```python
from build123d import *

# Parameters (mm, degrees)
SKETCH1_W               = 54.61
SKETCH1_H               = 47.244
SKETCH1_W_2             = 41.91
SKETCH1_H_2             = 21.844
BOSS_EXTRUDE1_DEPTH     = 5.08
SKETCH2_R               = 0.93599
CUT_EXTRUDE1_DEPTH      = 73.388217522
SKETCH10_W              = 14.41958
SKETCH10_H              = 19.49958
SKETCH10_R              = 0.635
BOSS_EXTRUDE4_DEPTH     = 5.08
SKETCH11_R              = 0.635
SKETCH11_W              = 3.302
SKETCH11_H              = 76.2
BOSS_EXTRUDE5_DEPTH     = 5.08
SKETCH12_W              = 60.452
SKETCH12_H              = 6.35
SKETCH12_W_2            = 59.182
CUT_EXTRUDE2_DEPTH      = 95.448366629
SKETCH13_W              = 7.0195552
SKETCH13_H              = 78.993394517
BOSS_EXTRUDE6_DEPTH     = 4.826
FILLET1_R               = 2.54
CUT_EXTRUDE3_DEPTH      = 95.448366629
SKETCH15_W              = 9.078627065
SKETCH15_H              = 34.544
BOSS_EXTRUDE7_DEPTH     = 5.08
SKETCH16_W              = 10.16
SKETCH16_H              = 12.7
BOSS_EXTRUDE8_DEPTH     = 10.16
SKETCH17_R              = 0.635
CUT_EXTRUDE4_DEPTH      = 71.364025147
SKETCH18_W              = 10.16
SKETCH18_H              = 6.35
BOSS_EXTRUDE9_DEPTH     = 12.76096
CUT_EXTRUDE5_DEPTH      = 73.410049688
CUT_EXTRUDE5_DEPTH_BACK = 73.410049688
SKETCH19_R              = 0.635
SKETCH20_W              = 10.16
SKETCH20_H              = 6.35
BOSS_EXTRUDE10_DEPTH    = 6.28904
CUT_EXTRUDE7_DEPTH      = 19.05


with BuildPart() as part:
    # Sketch1 → Boss-Extrude1 (new body)
    with BuildSketch(Plane.XY):
        with Locations((27.305, 23.622)):
            Rectangle(SKETCH1_W, SKETCH1_H)
        with Locations((27.305, 23.622)):
            Rectangle(SKETCH1_W_2, SKETCH1_H_2, mode=Mode.SUBTRACT)
    extrude(amount=BOSS_EXTRUDE1_DEPTH)

    # Sketch2 → Cut-Extrude1 (cut, through all)
    with BuildSketch(Plane.XY.offset(5.08)):
        with Locations((2.80543, 28.62199)):
            Circle(SKETCH2_R)
        with Locations((2.80543, 18.62201)):
            Circle(SKETCH2_R)
        with Locations((51.80457, 28.62199)):
            Circle(SKETCH2_R)
        with Locations((51.80457, 18.62201)):
            Circle(SKETCH2_R)
    extrude(amount=-CUT_EXTRUDE1_DEPTH, mode=Mode.SUBTRACT)

    # Sketch10 → Boss-Extrude4 (add)
    with BuildSketch(Plane.XY.offset(5.08)):
        with Locations((61.81979, 23.622)):
            Rectangle(SKETCH10_W, SKETCH10_H)
        with Locations((64.35979, 21.49221)):
            Circle(SKETCH10_R, mode=Mode.SUBTRACT)
        with Locations((64.35979, 25.75179)):
            Circle(SKETCH10_R, mode=Mode.SUBTRACT)
    extrude(amount=-BOSS_EXTRUDE4_DEPTH)

    # Sketch11 → Boss-Extrude5 (add)
    with BuildSketch(Plane.XY.offset(5.08)):
        Polygon((0, 47.244), (-5.842, 47.244), (-5.842, 64.262), (-15.748, 64.262), (-15.748, -17.018), (-4.572, -17.018), (-4.572, 0), (0, 0), align=None)
        with Locations(Location((-4.572, 21.49221, 0), (0, 0, 180))):
            Circle(SKETCH11_R, mode=Mode.SUBTRACT)
        with Locations(Location((-4.572, 25.75179, 0), (0, 0, 180))):
            Circle(SKETCH11_R, mode=Mode.SUBTRACT)
        with Locations((-10.795, 23.622)):
            Rectangle(SKETCH11_W, SKETCH11_H, mode=Mode.SUBTRACT)
    extrude(amount=-BOSS_EXTRUDE5_DEPTH)

    # Sketch12 → Cut-Extrude2 (cut, through all)
    with BuildSketch(Plane.XY.offset(5.08)):
        with Locations((24.384, 44.069)):
            Rectangle(SKETCH12_W, SKETCH12_H)
        with Locations((25.019, 3.175)):
            Rectangle(SKETCH12_W_2, SKETCH12_H)
    extrude(amount=-CUT_EXTRUDE2_DEPTH, mode=Mode.SUBTRACT)

    # Sketch13 → Boss-Extrude6 (add)
    with BuildSketch(Plane(origin=(0, 0, 0), x_dir=(-1, 0, 0), z_dir=(0, 0, -1))):
        with Locations((10.665198327, 23.388014827)):
            Rectangle(SKETCH13_W, SKETCH13_H)
    extrude(amount=-BOSS_EXTRUDE6_DEPTH)

    # Fillet1
    fillet1_edges = [part.edges().sort_by_distance(p)[0] for p in [
        (69.02958, 13.87221, 2.54),
        (54.61, 13.87221, 2.54),
        (54.61, 6.35, 2.54),
        (-4.572, 6.35, 2.54),
        (-4.572, -17.018, 2.54),
        (-15.748, -17.018, 2.54),
        (-15.748, 64.262, 2.54),
        (-5.842, 64.262, 2.54),
        (-5.842, 40.894, 2.54),
        (54.61, 40.894, 2.54),
        (54.61, 33.37179, 2.54),
        (69.02958, 33.37179, 2.54),
    ]]
    fillet(fillet1_edges, radius=FILLET1_R)

    # Sketch14 → Cut-Extrude3 (cut, through all)
    with BuildSketch(Plane.XY.offset(5.08)):
        Polygon((2.80543, 40.894), (-0.815942935, 40.894), (-0.815942935, 6.35), (2.80543, 6.35), (2.80543, -19.941776761), (-23.515321153, -19.941776761), (-23.515321153, 65.826532556), (2.80543, 65.826532556), align=None)
        Polygon((51.80457, 40.896870143), (51.80457, 65.826532556), (74.486186006, 65.826532556), (74.486186006, -19.941776761), (51.80457, -19.941776761), (52.07, 6.35), (54.61, 8.89), (54.61, 38.354), align=None)
    extrude(amount=-CUT_EXTRUDE3_DEPTH, mode=Mode.SUBTRACT)

    # Sketch15 → Boss-Extrude7 (add)
    with BuildSketch(Plane.XY.offset(5.08)):
        with Locations((-5.355256468, 23.622)):
            Rectangle(SKETCH15_W, SKETCH15_H)
        Polygon((51.807736495, 40.894), (54.61, 38.354), (54.61, 8.89), (52.07, 6.35), (64.50457, 6.35), (64.50457, 40.894), align=None)
    extrude(amount=-BOSS_EXTRUDE7_DEPTH)

    # Sketch16 → Boss-Extrude8 (add)
    with BuildSketch(Plane.XY.offset(5.08)):
        with Locations((-4.81457, 23.622)):
            Rectangle(SKETCH16_W, SKETCH16_H)
        with Locations((59.42457, 23.622)):
            Rectangle(SKETCH16_W, SKETCH16_H)
    extrude(amount=BOSS_EXTRUDE8_DEPTH)

    # Sketch17 → Cut-Extrude4 (cut, through all)
    with BuildSketch(Plane(origin=(0, 29.972, 0), x_dir=(1, 0, 0), z_dir=(0, 1, 0))):
        with Locations(Location((-4.81457, -10.16, 0), (0, 0, 180))):
            Circle(SKETCH17_R)
        with Locations(Location((59.42457, -10.16, 0), (0, 0, 180))):
            Circle(SKETCH17_R)
    extrude(amount=-CUT_EXTRUDE4_DEPTH, mode=Mode.SUBTRACT)

    # Sketch18 → Boss-Extrude9 (add)
    with BuildSketch(Plane.XY.offset(15.24)):
        with Locations((-4.81457, 20.447)):
            Rectangle(SKETCH18_W, SKETCH18_H)
        with Locations((59.42457, 26.797)):
            Rectangle(SKETCH18_W, SKETCH18_H)
    extrude(amount=BOSS_EXTRUDE9_DEPTH)

    # Sketch19 → Cut-Extrude5 (cut, two sides: drawn at the far end of the back side and taken through both)
    with BuildSketch(Plane(origin=(0, 23.622, 0), x_dir=(1, 0, 0), z_dir=(0, 1, 0)).offset(-CUT_EXTRUDE5_DEPTH_BACK)):
        with Locations(Location((-4.81457, -18.542, 0), (0, 0, 270))):
            Circle(SKETCH19_R)
        with Locations(Location((-4.81457, -24.69896, 0), (0, 0, 270))):
            Circle(SKETCH19_R)
        with Locations(Location((59.42457, -18.542, 0), (0, 0, 270))):
            Circle(SKETCH19_R)
        with Locations(Location((59.42457, -24.69896, 0), (0, 0, 270))):
            Circle(SKETCH19_R)
    extrude(amount=CUT_EXTRUDE5_DEPTH + CUT_EXTRUDE5_DEPTH_BACK, mode=Mode.SUBTRACT)

    # Sketch20 → Boss-Extrude10 (add)
    with BuildSketch(Plane.XY.offset(28.00096)):
        with Locations((-4.81457, 20.447)):
            Rectangle(SKETCH20_W, SKETCH20_H)
        with Locations((59.42457, 26.797)):
            Rectangle(SKETCH20_W, SKETCH20_H)
    extrude(amount=BOSS_EXTRUDE10_DEPTH)

    # Sketch22 → Cut-Extrude7 (cut)
    with BuildSketch(Plane.XY.offset(34.29)):
        Polygon((0.26543, 17.272), (-2.27457, 23.622), (0.26543, 23.622), align=None)
    extrude(amount=-CUT_EXTRUDE7_DEPTH, mode=Mode.SUBTRACT)


solid = part.part
```
The listing builds one solid part. Answer for the finished solid, in the listing's coordinates (mm). A direction names the side the tool comes from. Round coordinates to 2 decimals unless told otherwise and drop trailing zeros. Loops run counter-clockwise (first coordinate to the right, second up) from the corner with the lowest first, then second, coordinate; pieces in that order, holes last. Notation, with made-up numbers: (-13.75, -32.75) - (-3.75, -32.75) arc R26 cw to (-3.75, -13.75) - close; hole circle Ø11 at (40, -14). An arc over 180 degrees is marked (long way). Return JSON: item names as keys, results as strings. Group by question number.
1. Consider probe 1 along Y at (x, z) = (10, 5); probe 2 along X at (y, z) = (20, 7.5); probe 3 along X at (y, z) = (31, 3). Determine where each line is inside the solid, lowest interval first.
2. The part is cut by section B-B on y = 22. Determine the outline of the cut face in (x, z) (3 decimals).
3. The part is cut by section C-C on z = 17. Determine the outline of the cut face in (x, y), then the cut area to 3 significant figures.
4. The part is cut by section D-D on x = -3. Determine the outline of the cut face in (y, z).
5. The part is cut by section A-A on x = 13.5. Determine the outline of the cut face in (y, z), then the cut area to 3 significant figures.
6. Each of these flat-tipped pins is pushed along its axis until it touches: P1, Ø10, axis at x = 45, y = 29.5, coming from the +Z side; P2, Ø8, axis at x = 61.5, z = 29, coming from the -Y side; P3, Ø1.5, axis at x = 59.42, z = 10.16, coming from the +Y side. Where does it stop, or does it pass through?
7. Which of the six approach directions +Z, -Z, +X, -X, +Y, -Y give full straight-line access (tool end or side, diameter ignored) to faces 5 (the flat face through (-5, 29.972, 11)), 6 (the flat face through (60.5, 23.622, 24.6)), 7 (the flat face through (-6, 23.622, 25)), 8 (the flat face through (-0.987, 20.403, 24.898)), 9 (the flat face through (27, 12.7, 3))?
8. The mould has two halves that part along X. Classify faces 1 (the flat face through (-9.895, 22, 11)), 2 (the flat face through (64.505, 25, 12)), 3 (the flat face through (-5, 27, 15.24)), 4 (the cylindrical face through (2.6, 17.71, 2.58)): pulls with the +X half, pulls with the -X half, needs draft (parallel to the pull), parting line crosses it, or undercut.
Resolved:
{
 "1": {"probe 1": "y = 6.35 to 12.7, 34.54 to 40.89", "probe 2": "x = -9.89 to 0.27, 54.34 to 64.5", "probe 3": "x = -9.89 to 6.35, 48.26 to 64.5"},
 "2": {"outline": "(-9.895, 0) - (6.35, 0) - (6.35, 5.08) - (0.265, 5.08) - (0.265, 15.24) - (-1.626, 15.24) - (-1.626, 34.29) - (-9.895, 34.29) - close; (48.26, 0) - (64.505, 0) - (64.505, 15.24) - (54.345, 15.24) - (54.345, 5.08) - (48.26, 5.08) - close; hole circle Ø1.27 at (-4.815, 10.16); hole circle Ø1.27 at (-4.815, 18.542); hole circle Ø1.27 at (-4.815, 24.699); hole circle Ø1.27 at (59.425, 10.16)"},
 "3": {"outline": "(-9.89, 17.27) - (0.27, 17.27) - (-2.27, 23.62) - (-9.89, 23.62) - close; (54.34, 23.62) - (64.5, 23.62) - (64.5, 29.97) - (54.34, 29.97) - close", "area": "121 mm²"},
 "4": {"outline": "(6.35, 0) - (40.89, 0) - (40.89, 5.08) - (29.97, 5.08) - (29.97, 15.24) - (23.62, 15.24) - (23.62, 34.29) - (17.27, 34.29) - (17.27, 5.08) - (6.35, 5.08) - close"},
 "5": {"outline": "(6.35, 0) - (12.7, 0) - (12.7, 5.08) - (6.35, 5.08) - close; (34.54, 0) - (40.89, 0) - (40.89, 5.08) - (34.54, 5.08) - close", "area": "64.5 mm²"},
 "6": {"P1": "stops at z = 5.08", "P2": "stops at y = 23.62", "P3": "stops at y = 29.97"},
 "7": {"face 5": "+Z, +X, -X, +Y", "face 6": "+Z, +X, -Y", "face 7": "+Z, -X, +Y", "face 8": "+Z, +X, +Y", "face 9": "+Z, -Z"},
 "8": {"face 1": "pulls with the -X half", "face 2": "pulls with the +X half", "face 3": "needs draft", "face 4": "undercut"}
}
